```python
from build123d import *

# Parameters (mm, degrees)
SKETCH2_W           = 120
SKETCH2_H           = 120
SKETCH2_W_2         = 100
SKETCH2_H_2         = 100
BOSS_EXTRUDE1_DEPTH = 100
SKETCH3_W           = 120
SKETCH3_H           = 120
BOSS_EXTRUDE2_DEPTH = 20
SKETCH4_W           = 120
SKETCH4_H           = 120
BOSS_EXTRUDE3_DEPTH = 20
SKETCH5_W           = 75
SKETCH5_H           = 20
CUT_EXTRUDE1_DEPTH  = 150


with BuildPart() as part:
    # Sketch2 → Boss-Extrude1 (new body)
    with BuildSketch(Plane(origin=(0, 0, 0), x_dir=(1, 0, 0), z_dir=(0, 1, 0))):
        Rectangle(SKETCH2_W, SKETCH2_H)
        Rectangle(SKETCH2_W_2, SKETCH2_H_2, mode=Mode.SUBTRACT)
    extrude(amount=BOSS_EXTRUDE1_DEPTH)

    # Sketch3 → Boss-Extrude2 (add)
    with BuildSketch(Plane.XZ):
        Rectangle(SKETCH3_W, SKETCH3_H)
    extrude(amount=BOSS_EXTRUDE2_DEPTH)

    # Sketch4 → Boss-Extrude3 (add)
    with BuildSketch(Plane(origin=(0, 100, 0), x_dir=(1, 0, 0), z_dir=(0, 1, 0))):
        Rectangle(SKETCH4_W, SKETCH4_H)
    extrude(amount=BOSS_EXTRUDE3_DEPTH)

    # Sketch5 → Cut-Extrude1 (cut)
    with BuildSketch(Plane(origin=(0, 120, 0), x_dir=(1, 0, 0), z_dir=(0, 1, 0))):
        with Locations((22.5, 0)):
            Rectangle(SKETCH5_W, SKETCH5_H)
    extrude(amount=-CUT_EXTRUDE1_DEPTH, mode=Mode.SUBTRACT)


solid = part.part
```
The model under review builds one solid part; all positions refer to its coordinate system, in mm. A direction names the side the tool comes from. Round coordinates to 2 decimals unless told otherwise and drop trailing zeros. Loops run counter-clockwise (first coordinate to the right, second up) from the corner with the lowest first, then second, coordinate; pieces in that order, holes last. Notation, with made-up numbers: (70.5, 83.25) - (79.5, 83.25) arc R23 cw to (79.5, 119.25) - close; hole circle Ø2 at (-4.75, 47.25). An arc over 180 degrees is marked (long way). Use a Markdown table: item, result. Add a question column.
Q1. Add section A-A (x = 24). State the section outline as (y, z) points.
Q2. Add section B-B (z = -42). State the section outline as (x, y) points, plus the area to 3 significant figures.
Q3. Machinability: for faces 1 (the face through (-15, 110, 0)), 2 (the face through (-1, 49, -60)), 3 (the face through (-50, 49, 1)), which of the approach directions +Z, -Z, +X, -X, +Y, -Y give a long, thin tool a straight path to every point of the face, cutting with its end or side? Answer none if there is none.
Q4. For probe 1 along Z at (x, y) = (-24, 34); probe 2 along Y at (x, z) = (32.5, -40.5), list the stretches that pass through material, from the lowest coordinate up.
Q5. Add section C-C (y = 109). State the section outline as (x, z) points.
Q6. Add section D-D (z = -7.5). State the section outline as (x, y) points, plus the area to 3 significant figures.
Q7. Insertion check: pin 1 Ø6 at (y, z) = (-13.5, 4.5) entering from +X. The pin has a flat end and moves straight along its axis. Give the tip position at first contact, or say it passes through.
Q8. The part is to be moulded in two halves that separate along Y. For faces 4 (the face through (-1, 120, -14)), 5 (the face through (-1, 49, 50)), 6 (the face through (53, 56, -10)), 7 (the face through (-1, -20, 14)), say which applies: pulls with the +Y half, pulls with the -Y half, needs draft (parallel to the pull), parting line crosses it, or undercut.
Worked answers:
| question | item | result |
|---|---|---|
| 1 | outline | (-20, -60) - (120, -60) - (120, -10) - (100, -10) - (100, -50) - (0, -50) - (0, -10) - (-20, -10) - close; (-20, 10) - (0, 10) - (0, 50) - (100, 50) - (100, 10) - (120, 10) - (120, 60) - (-20, 60) - close |
| 2 | outline | (-60, -20) - (60, -20) - (60, 120) - (-60, 120) - close; hole (-50, 0) - (50, 0) - (50, 100) - (-50, 100) - close |
| 2 | area | 6,800 mm² |
| 3 | face 1 | +X, +Y, -Y |
| 3 | face 2 | -Z, +X, -X, +Y, -Y |
| 3 | face 3 | none |
| 4 | probe 1 | -60 to -50, 50 to 60 |
| 4 | probe 2 | -20 to 0, 100 to 120 |
| 5 | outline | (-60, -60) - (60, -60) - (60, -10) - (-15, -10) - (-15, 10) - (60, 10) - (60, 60) - (-60, 60) - close |
| 6 | outline | (-60, -20) - (-15, -20) - (-15, 0) - (-50, 0) - (-50, 100) - (-15, 100) - (-15, 120) - (-60, 120) - close |
| 6 | area | 2,800 mm² |
| 7 | pin 1 | x = -15 |
| 8 | face 4 | pulls with the +Y half |
| 8 | face 5 | undercut |
| 8 | face 6 | needs draft |
| 8 | face 7 | pulls with the -Y half |
